from build123d import *

# Parameters (mm, degrees)
SKETCH1_R                        = 18.5
BOSS_EXTRUDE1_DEPTH              = 19
SKETCH4_R                        = 6
BOSS_EXTRUDE4_DEPTH              = 6
CUT_EXTRUDE2_DEPTH               = 1
TALADRO_DE_MARGEN_PARA_M31_D     = 3.4
TALADRO_DE_MARGEN_PARA_M31_DEPTH = 6
TALADRO_DE_MARGEN_PARA_M31_TIP   = 1.021463052
CROQUIS1_R                       = 18
CORTAR_EXTRUIR2_DEPTH            = 12
CORTAR_EXTRUIR3_REACH            = 27
CROQUIS2_R                       = 3
CROQUIS2_R_2                     = 1.7
CROQUIS3_R                       = 18
SALIENTE_EXTRUIR1_DEPTH          = 0.5
SKETCH11_R                       = 2
CUT_EXTRUDE3_DEPTH               = 10
SKETCH12_W                       = 12.5
SKETCH12_H                       = 1.5
CUT_EXTRUDE4_DEPTH               = 0.15
SKETCH13_R                       = 6
CUT_EXTRUDE5_DEPTH               = 10
SKETCH14_R                       = 2.25
SKETCH14_R_2                     = 2
BOSS_EXTRUDE5_DEPTH              = 1


with BuildPart() as part:
    # Sketch1 → Boss-Extrude1 (new body)
    with BuildSketch(Plane.XY):
        Circle(SKETCH1_R)
    extrude(amount=BOSS_EXTRUDE1_DEPTH)

    # Sketch4 → Boss-Extrude4 (add)
    with BuildSketch(Plane.XY.offset(19)):
        with Locations((0, 7)):
            Circle(SKETCH4_R)
    extrude(amount=BOSS_EXTRUDE4_DEPTH)

    # Sketch8 → Cut-Extrude2 (cut)
    with BuildSketch(Plane.XY.offset(19)):
        with BuildLine():
            ThreePointArc((7.635768375, 9.386428571), (0, -12.1), (-7.635768375, 9.386428571))
            ThreePointArc((-7.635768375, 9.386428571), (0, -1), (7.635768375, 9.386428571))
        make_face()
    extrude(amount=-CUT_EXTRUDE2_DEPTH, mode=Mode.SUBTRACT)

    # Taladro de margen para M31
    with Locations(Plane.XY.offset(19)):
        with Locations((7.65, -13.250188678), (-7.65, -13.250188678), (-15.3, 0), (-7.65, 13.250188678), (15.3, 0), (7.65, 13.250188678)):
            Hole(TALADRO_DE_MARGEN_PARA_M31_D / 2, depth=TALADRO_DE_MARGEN_PARA_M31_DEPTH)
            with Locations((0, 0, -(TALADRO_DE_MARGEN_PARA_M31_DEPTH + TALADRO_DE_MARGEN_PARA_M31_TIP / 2))):  # 118° drill point
                Cone(0, TALADRO_DE_MARGEN_PARA_M31_D / 2, TALADRO_DE_MARGEN_PARA_M31_TIP, mode=Mode.SUBTRACT)

    # Croquis1 → Cortar-Extruir2 (cut)
    with BuildSketch(Plane(origin=(0, 0, 0), x_dir=(-1, 0, 0), z_dir=(0, 0, -1))):
        Circle(CROQUIS1_R)
    extrude(amount=-CORTAR_EXTRUIR2_DEPTH, mode=Mode.SUBTRACT)

    # Croquis2 → Cortar-Extruir3 (cut, up to next)
    with BuildSketch(Plane.XY.offset(25), mode=Mode.PRIVATE) as cortar_extruir3_sk1:
        with Locations((0, 7)):
            Circle(CROQUIS2_R)
    cortar_extruir3_tool1 = extrude(cortar_extruir3_sk1.sketch, amount=-CORTAR_EXTRUIR3_REACH, mode=Mode.PRIVATE) & part.part
    add(cortar_extruir3_tool1.solids().sort_by_distance((0, 7, 25))[0], mode=Mode.SUBTRACT)
    # Croquis2 → Cortar-Extruir3 (cut, up to next)
    with BuildSketch(Plane.XY.offset(25), mode=Mode.PRIVATE) as cortar_extruir3_sk2:
        with Locations((7.65, 13.250188678)):
            Circle(CROQUIS2_R_2)
    cortar_extruir3_tool2 = extrude(cortar_extruir3_sk2.sketch, amount=-CORTAR_EXTRUIR3_REACH, mode=Mode.PRIVATE) & part.part
    add(cortar_extruir3_tool2.solids().sort_by_distance((7.65, 13.250189, 25))[0], mode=Mode.SUBTRACT)

    # Croquis3 → Saliente-Extruir1 (add)
    with BuildSketch(Plane(origin=(0, 0, 0), x_dir=(-1, 0, 0), z_dir=(0, 0, -1))):
        Circle(CROQUIS3_R)
    extrude(amount=-SALIENTE_EXTRUIR1_DEPTH)

    # Sketch11 → Cut-Extrude3 (cut)
    with BuildSketch(Plane(origin=(0, 0, 0), x_dir=(-1, 0, 0), z_dir=(0, 0, -1))):
        Circle(SKETCH11_R)
    extrude(amount=-CUT_EXTRUDE3_DEPTH, mode=Mode.SUBTRACT)

    # Sketch12 → Cut-Extrude4 (cut)
    with BuildSketch(Plane(origin=(0, 0, 0), x_dir=(-1, 0, 0), z_dir=(0, 0, -1))):
        with Locations((0, -15)):
            Rectangle(SKETCH12_W, SKETCH12_H)
    extrude(amount=-CUT_EXTRUDE4_DEPTH, mode=Mode.SUBTRACT)

    # Sketch13 → Cut-Extrude5 (cut)
    with BuildSketch(Plane(origin=(0, 0, 0), x_dir=(-1, 0, 0), z_dir=(0, 0, -1))):
        Circle(SKETCH13_R)
    extrude(amount=-CUT_EXTRUDE5_DEPTH, mode=Mode.SUBTRACT)

    # Sketch14 → Boss-Extrude5 (add)
    with BuildSketch(Plane(origin=(0, 0, 12), x_dir=(-1, 0, 0), z_dir=(0, 0, -1))):
        with Locations((0, -5.15)):
            Circle(SKETCH14_R)
        with Locations((0, -5.15)):
            Circle(SKETCH14_R_2, mode=Mode.SUBTRACT)
    extrude(amount=BOSS_EXTRUDE5_DEPTH)


solid = part.part
Source: CAD feature listing. Evaluate the final solid. Frame: model axes, mm. A direction names the side the tool comes from. Round coordinates to 2 decimals unless told otherwise and drop trailing zeros. Write each loop counter-clockwise with the first axis right and the second up, starting at its lowest first coordinate (ties: lowest second). Pieces come first, ordered by that corner, then holes. Notation, with made-up numbers: (85.25, -21) - (107.25, -21) arc R13 cw to (107.25, 3) - close; hole circle Ø9 at (-28.5, 85). An arc over 180 degrees is marked (long way). Use CSV: the item, a comma, the result in double quotes. Start each with the question number.
(1) Mould query, pull axis X, two halves, no side actions, for faces 5 (the face through (-7.34, -13.153, 12.174)), 6 (the face through (-0.78, 12.95, 21.96)), 7 (the face through (14.98, 0.01, 12.17)), 8 (the face through (0, 0, 19)). Classes: pulls with the +X half, pulls with the -X half, needs draft (parallel to the pull), parting line crosses it, or undercut.
(2) Cut plane D-D, the plane y = -10.5. Return loops of the section in (x, z).
(3) Cut plane A-A, the plane y = 5.5. Return loops of the section in (x, z).
(4) First-contact query: pin 1 Ø5 at (x, y) = (0, -4) entering from -Z; pin 2 Ø5 at (x, z) = (1.5, 7.5) entering from +Y; pin 3 Ø10 at (y, z) = (-7.5, 18) entering from -X; pin 4 Ø0.8 at (x, y) = (-1.5, -15) entering from -Z. Flat tips, straight axial feed; report the tip coordinate or a pass-through.
(5) Cut plane B-B, the plane z = 16. Return loops of the section in (x, y), and give its area (3 significant figures).
(6) Cut plane C-C, the plane z = 20. Return loops of the section in (x, y), and give its area (3 significant figures).
(7) Material intervals for probe 1 along Z at (x, y) = (5, 8.5); probe 2 along Y at (x, z) = (7.65, 17.4); probe 3 along Z at (x, y) = (11, -11.5), sorted ascending. Write a range as [from, to].
(8) Set-up query: faces 1 (the face through (0, -8, 0.5)), 2 (the face through (5.994, 0.264, 0.246)), 3 (the face through (1, 10, 25)), 4 (the face through (13.73, -0.65, 15.96)). Return all of +Z, -Z, +X, -X, +Y, -Y with unobstructed straight access to the full face (end or side cutting, diameter ignored); none if empty.
Geometry says:
1,face 5,"undercut"
1,face 6,"parting line crosses it"
1,face 7,"undercut"
1,face 8,"needs draft"
2,outline,"(-15.23, 0) - (15.23, 0) - (15.23, 19) - (6.01, 19) - (6.01, 18) - (-6.01, 18) - (-6.01, 19) - (-15.23, 19) - close; hole (-14.62, 0.5) - (14.62, 0.5) - (14.62, 12) - (-14.62, 12) - close"
3,outline,"(-17.66, 0) - (-2.4, 0) - (-2.4, 0.5) - (-17.14, 0.5) - (-17.14, 12) - (-2.6, 12) - (-2.6, 25) - (-5.81, 25) - (-5.81, 19) - (-7.86, 19) - (-7.86, 18) - (-10.78, 18) - (-10.78, 19) - (-17.66, 19) - close; (2.4, 0) - (17.66, 0) - (17.66, 19) - (10.78, 19) - (10.78, 18) - (7.86, 18) - (7.86, 19) - (5.81, 19) - (5.81, 25) - (2.6, 25) - (2.6, 12) - (17.14, 12) - (17.14, 0.5) - (2.4, 0.5) - close"
4,pin 1,"z = 0"
4,pin 2,"y = 18.5"
4,pin 3,"x = -18.33"
4,pin 4,"z = 0.15"
5,outline,"circle Ø37 at (0, 0); hole circle Ø3.4 at (-15.3, 0); hole circle Ø3.4 at (-7.65, -13.25); hole circle Ø3.4 at (-7.65, 13.25); hole circle Ø6 at (0, 7); hole circle Ø3.4 at (7.65, -13.25); hole circle Ø3.4 at (7.65, 13.25); hole circle Ø3.4 at (15.3, 0)"
5,area,"992 mm²"
6,outline,"circle Ø12 at (0, 7); hole circle Ø6 at (0, 7)"
6,area,"84.8 mm²"
7,probe 1,"[0, 0.5], [12, 25]"
7,probe 2,"[-16.84, -14.95], [-11.55, 11.55], [14.95, 16.84]"
7,probe 3,"[0, 0.5], [12, 19]"
8,face 1,"none"
8,face 2,"-Z"
8,face 3,"+Z, +X, -X, +Y, -Y"
8,face 4,"+Z"
